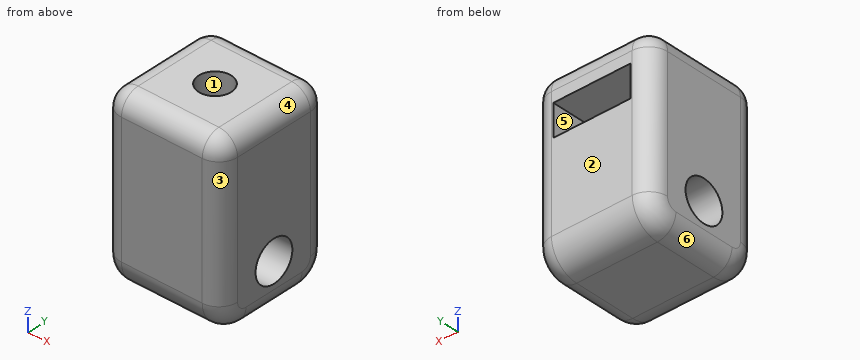
```python
from build123d import *

# Parameters (mm, degrees)
SKETCH1_W           = 50.8
SKETCH1_H           = 19.05
BOSS_EXTRUDE1_DEPTH = 12.7
SKETCH2_R           = 2.2
CUT_EXTRUDE1_DEPTH  = 56.72102386
SKETCH4_R           = 1.7525
CUT_EXTRUDE3_DEPTH  = 3.4
CUT_EXTRUDE4_START  = -3.4
SKETCH4_3_R         = 1.7525
CUT_EXTRUDE4_DEPTH  = 3
CUT_EXTRUDE5_REACH  = 56.717
SKETCH4_4_R         = 1.7525
CUT_EXTRUDE6_REACH  = 57.721
SKETCH5_W           = 38.1
SKETCH5_H           = 19.05
FILLET1_R           = 3
FILLET2_R           = 2
FILLET3_R           = 2


with BuildPart() as part:
    # Sketch1 → Boss-Extrude1 (new body)
    with BuildSketch(Plane(origin=(0, 0, 0), x_dir=(1, 0, 0), z_dir=(0, 1, 0))):
        with Locations((-25.4, -9.525)):
            Rectangle(SKETCH1_W, SKETCH1_H)
    extrude(amount=BOSS_EXTRUDE1_DEPTH)

    # Sketch2 → Cut-Extrude1 (cut, through all)
    with BuildSketch(Plane.ZY.offset(50.8)):
        with Locations((4.7625, 6.35)):
            Circle(SKETCH2_R)
    extrude(amount=-CUT_EXTRUDE1_DEPTH, mode=Mode.SUBTRACT)

    # Sketch4 → Cut-Extrude3 (cut)
    # profile 1 of 9: a face of its own
    with BuildSketch(Plane.XY.offset(15.875)):
        Polygon((-40.3, 12.7), (-40.3, 8.746003617), (-44.45, 11.142007234), (-48.6, 8.746003617), (-48.6, 12.7), align=None)
    # profile 2 of 9: a face of its own
    with BuildSketch(Plane.XY.offset(15.875)):
        Polygon((-48.6, 8.746003617), (-48.6, 3.953996383), (-44.45, 1.557992766), (-40.3, 3.953996383), (-40.3, 8.746003617), (-44.45, 11.142007234), align=None)
        with Locations((-44.45, 6.35)):
            Circle(SKETCH4_R, mode=Mode.SUBTRACT)
    # profile 3 of 9: a face of its own
    with BuildSketch(Plane.XY.offset(15.875)):
        Polygon((-35.9, 12.7), (-27.6, 12.7), (-27.6, 8.746003617), (-27.6, 3.953996383), (-31.75, 1.557992766), (-35.9, 3.953996383), (-35.9, 8.746003617), align=None)
        with Locations((-31.75, 6.35)):
            Circle(SKETCH4_R, mode=Mode.SUBTRACT)
    # profile 4 of 9: a face of its own
    with BuildSketch(Plane.XY.offset(15.875)):
        with Locations((-31.75, 6.35)):
            Circle(SKETCH4_R)
    # profile 5 of 9: a face of its own
    with BuildSketch(Plane.XY.offset(15.875)):
        with Locations((-44.45, 6.35)):
            Circle(SKETCH4_R)
    # profile 6 of 9: a face of its own
    with BuildSketch(Plane.XY.offset(15.875)):
        Polygon((-23.2, 12.7), (-14.9, 12.7), (-14.9, 8.746003617), (-14.9, 3.953996383), (-19.05, 1.557992766), (-23.2, 3.953996383), (-23.2, 8.746003617), align=None)
        with Locations((-19.05, 6.35)):
            Circle(SKETCH4_R, mode=Mode.SUBTRACT)
    # profile 7 of 9: a face of its own
    with BuildSketch(Plane.XY.offset(15.875)):
        with Locations((-19.05, 6.35)):
            Circle(SKETCH4_R)
    # profile 8 of 9: a face of its own
    with BuildSketch(Plane.XY.offset(15.875)):
        Polygon((-10.5, 12.7), (-2.2, 12.7), (-2.2, 8.746003617), (-2.2, 3.953996383), (-6.35, 1.557992766), (-10.5, 3.953996383), (-10.5, 8.746003617), align=None)
        with Locations((-6.35, 6.35)):
            Circle(SKETCH4_R, mode=Mode.SUBTRACT)
    # profile 9 of 9: a face of its own
    with BuildSketch(Plane.XY.offset(15.875)):
        with Locations((-6.35, 6.35)):
            Circle(SKETCH4_R)
    extrude(amount=-CUT_EXTRUDE3_DEPTH, mode=Mode.SUBTRACT)

    # Sketch4<3> → Cut-Extrude4 (cut)
    with BuildSketch(Plane.XY.offset(15.875).offset(CUT_EXTRUDE4_START)):
        with Locations((-44.45, 6.35)):
            Circle(SKETCH4_3_R)
        with Locations((-31.75, 6.35)):
            Circle(SKETCH4_3_R)
        with Locations((-19.05, 6.35)):
            Circle(SKETCH4_3_R)
        with Locations((-6.35, 6.35)):
            Circle(SKETCH4_3_R)
    extrude(amount=-CUT_EXTRUDE4_DEPTH, mode=Mode.SUBTRACT)

    # Sketch4<4> → Cut-Extrude5 (cut, up to next)
    with BuildSketch(Plane.XY.offset(15.875), mode=Mode.PRIVATE) as cut_extrude5_sk1:
        with Locations((-44.45, 6.35)):
            Circle(SKETCH4_4_R)
    cut_extrude5_tool1 = extrude(cut_extrude5_sk1.sketch, amount=CUT_EXTRUDE5_REACH, mode=Mode.PRIVATE) & part.part
    # Sketch4<4> → Cut-Extrude5 (cut, up to next)
    with BuildSketch(Plane.XY.offset(15.875), mode=Mode.PRIVATE) as cut_extrude5_sk2:
        with Locations((-31.75, 6.35)):
            Circle(SKETCH4_4_R)
    cut_extrude5_tool2 = extrude(cut_extrude5_sk2.sketch, amount=CUT_EXTRUDE5_REACH, mode=Mode.PRIVATE) & part.part
    # Sketch4<4> → Cut-Extrude5 (cut, up to next)
    with BuildSketch(Plane.XY.offset(15.875), mode=Mode.PRIVATE) as cut_extrude5_sk3:
        with Locations((-19.05, 6.35)):
            Circle(SKETCH4_4_R)
    cut_extrude5_tool3 = extrude(cut_extrude5_sk3.sketch, amount=CUT_EXTRUDE5_REACH, mode=Mode.PRIVATE) & part.part
    # Sketch4<4> → Cut-Extrude5 (cut, up to next)
    with BuildSketch(Plane.XY.offset(15.875), mode=Mode.PRIVATE) as cut_extrude5_sk4:
        with Locations((-6.35, 6.35)):
            Circle(SKETCH4_4_R)
    cut_extrude5_tool4 = extrude(cut_extrude5_sk4.sketch, amount=CUT_EXTRUDE5_REACH, mode=Mode.PRIVATE) & part.part
    add(cut_extrude5_tool1.solids().sort_by_distance((-44.45, 6.35, 15.875))[0], mode=Mode.SUBTRACT)
    add(cut_extrude5_tool2.solids().sort_by_distance((-31.75, 6.35, 15.875))[0], mode=Mode.SUBTRACT)
    add(cut_extrude5_tool3.solids().sort_by_distance((-19.05, 6.35, 15.875))[0], mode=Mode.SUBTRACT)
    add(cut_extrude5_tool4.solids().sort_by_distance((-6.35, 6.35, 15.875))[0], mode=Mode.SUBTRACT)

    # Sketch5 → Cut-Extrude6 (cut, up to next)
    with BuildSketch(Plane(origin=(0, 12.7, 0), x_dir=(1, 0, 0), z_dir=(0, 1, 0)), mode=Mode.PRIVATE) as cut_extrude6_sk1:
        with Locations((-19.05, -9.525)):
            Rectangle(SKETCH5_W, SKETCH5_H)
    cut_extrude6_tool1 = extrude(cut_extrude6_sk1.sketch, amount=-CUT_EXTRUDE6_REACH, mode=Mode.PRIVATE) & part.part
    add(cut_extrude6_tool1.solids().sort_by_distance((-19.05, 12.7, 9.525))[0], mode=Mode.SUBTRACT)

    # Fillet1
    fillet1_edges = [part.edges().sort_by_distance(p)[0] for p in [
        (-44.45, 0, 0),
        (-44.45, 12.7, 0),
    ]]
    fillet(fillet1_edges, radius=FILLET1_R)

    # Fillet2
    fillet2_edges = [part.edges().sort_by_distance(p)[0] for p in [
        (-44.45, 12.7, 19.05),
        (-44.45, 0, 19.05),
    ]]
    fillet(fillet2_edges, radius=FILLET2_R)

    # Fillet3
    fillet3_edges = [part.edges().sort_by_distance(p)[0] for p in [
        (-38.1, 6.35, 0),
        (-50.8, 6.35, 0),
        (-50.8, 0, 10.025),
        (-50.8, 12.7, 10.025),
        (-50.8, 11.821320344, 0.878679656),
        (-50.8, 0.878679656, 0.878679656),
        (-38.1, 0, 10.025),
        (-38.1, 12.7, 10.025),
        (-38.1, 11.821320344, 0.878679656),
        (-38.1, 0.878679656, 0.878679656),
        (-38.1, 6.35, 19.05),
        (-50.8, 6.35, 19.05),
        (-38.1, 12.114213562, 18.464213562),
        (-38.1, 0.585786438, 18.464213562),
        (-50.8, 12.114213562, 18.464213562),
        (-50.8, 0.585786438, 18.464213562),
    ]]
    fillet(fillet3_edges, radius=FILLET3_R)


solid = part.part
```
Work out the finished part from the listing and answer in its coordinate system (mm). Face numbers are marked on the shaded views. A direction names the side the tool comes from. Round coordinates to 2 decimals unless told otherwise and drop trailing zeros. Loops run counter-clockwise (first coordinate to the right, second up) from the corner with the lowest first, then second, coordinate; pieces in that order, holes last.
(1) The part is cut by section C-C, the plane z = 6.75. Give the vertices of the cut face in (x, y).
Computed values:
outline: (-50.8, 2) arc R2 ccw to (-48.8, 0) - (-40.1, 0) arc R2 ccw to (-38.1, 2) - (-38.1, 5.41) - (-50.8, 5.41) - close; (-50.8, 7.29) - (-38.1, 7.29) - (-38.1, 10.7) arc R2 ccw to (-40.1, 12.7) - (-48.8, 12.7) arc R2 ccw to (-50.8, 10.7) - close
(2) The mould has two halves that part along Y. Classify the marked faces 1, 2, 3 and 4: pulls with the +Y half, pulls with the -Y half, needs draft (parallel to the pull), parting line crosses it, or undercut.
Computed values:
face 1: undercut
face 2: pulls with the +Y half
face 3: pulls with the -Y half
face 4: needs draft
(3) The part is cut by section A-A, the plane x = -44.75. Give the number of separate pieces and of enclosed holes in the cut face, and give its area (3 significant figures).
Computed values:
separate pieces: 2
enclosed holes: 1
area: 163 mm2
(4) Find the intervals of material crossed by L1, parallel to Y at x = -44.45, z = 11.75; L2, parallel to Z at x = -43, y = 5 (3 decimals); L3, parallel to X at y = 6.75, z = 14.25, in increasing order.
Computed values:
L1: y = 0 to 4.6, 8.1 to 12.7
L2: z = 0 to 3.025, 6.5 to 12.475, 15.875 to 19.05
L3: x = -50.8 to -48.6, -40.3 to -38.1
(5) The part is cut by section D-D, the plane y = 5.5. Give the vertices of the cut face in (x, z) (3 decimals).
Computed values:
outline: (-50.8, 2) arc R2 ccw to (-48.8, 0) - (-40.1, 0) arc R2 ccw to (-38.1, 2) - (-38.1, 2.733) - (-50.8, 2.733) - close; (-50.8, 6.792) - (-38.1, 6.792) - (-38.1, 17.05) arc R2 ccw to (-40.1, 19.05) - (-42.917, 19.05) - (-42.917, 15.875) - (-40.3, 15.875) - (-40.3, 12.475) - (-42.917, 12.475) - (-42.917, 9.475) - (-45.983, 9.475) - (-45.983, 12.475) - (-48.6, 12.475) - (-48.6, 15.875) - (-45.983, 15.875) - (-45.983, 19.05) - (-48.8, 19.05) arc R2 ccw to (-50.8, 17.05) - close
(6) For the marked faces 5 and 6, determine the directions among +Z, -Z, +X, -X, +Y, -Y from which every point of the face is accessible in a straight line to the end or side of a thin tool.
Computed values:
face 5: +Y
face 6: -Z, -X, +Y, -Y
(7) This flat-tipped pin is pushed along its axis until it touches: P1, Ø1, axis at x = -45.5, y = 2, coming from the -Z side. Where does it stop, or does it pass through?
Computed values:
P1: stops at z = 0.04
(8) The part is cut by section B-B, the plane y = 9. Give the vertices of the cut face in (x, z) (3 decimals), and give its area (3 significant figures).
Computed values:
outline: (-50.8, 2) arc R2 ccw to (-48.8, 0) - (-40.1, 0) arc R2 ccw to (-38.1, 2) - (-38.1, 17.05) arc R2 ccw to (-40.1, 19.05) - (-48.8, 19.05) arc R2 ccw to (-50.8, 17.05) - close; hole (-48.6, 12.475) - (-40.3, 12.475) - (-40.3, 15.875) - (-48.6, 15.875) - close
area: 210 mm2
